Check sheet for the modelled part. Datum: model origin and axes. Units: mm. Face numbers are marked on the shaded views. A direction names the side the tool comes from. Give positions to 0.01 mm unless a question says otherwise; leave off trailing zeros. Order: outer loops, then holes, each group sorted by start corner. A loop starts at its lowest first (then second) coordinate and runs counter-clockwise, first axis right, second up.
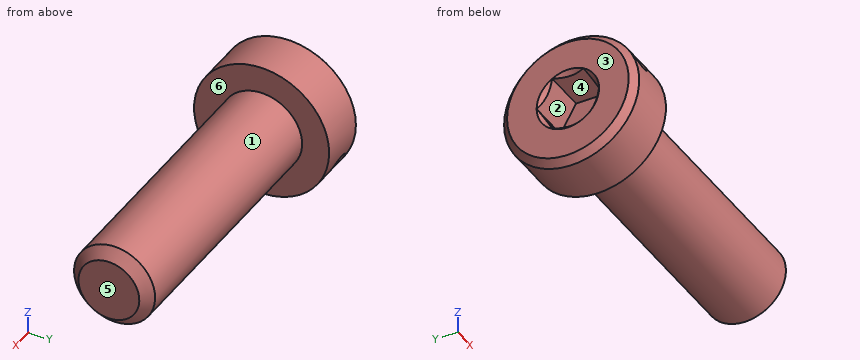
from build123d import *

# Parameters (mm, degrees)
SKETCH2_R               = 3
BOSS_EXTRUDE1_DEPTH     = 20
CHAMFER1_SIZE           = 0.75
CUT_EXTRUDE1_DEPTH      = 3.12
CUT_EXTRUDE3_DEPTH      = 17.652942925
CUT_EXTRUDE3_DEPTH_BACK = 17.652942925
SKETCH9_R               = 0.79375


with BuildPart() as part:
    # Sketch2 → Boss-Extrude1 (new body)
    with BuildSketch(Plane(origin=(10, 0, 0), x_dir=(0, 0, -1), z_dir=(1, 0, 0))):
        Circle(SKETCH2_R)
    extrude(amount=-BOSS_EXTRUDE1_DEPTH)

    # Chamfer1
    chamfer1_edges = [part.edges().sort_by_distance(p)[0] for p in [
        (10, 0, 3),
    ]]
    chamfer(chamfer1_edges, length=CHAMFER1_SIZE)

    # Sketch6 → Revolve1 (revolve)
    with BuildSketch(Plane.XY):
        Polygon((-13.5, 5), (-14, 4.5), (-14, 0), (-10, 0), (-10, 5), align=None)
    revolve(axis=Axis((-10, 0, 0), (-1, 0, 0)))

    # Sketch4 → Cut-Extrude1 (cut)
    with BuildSketch(Plane(origin=(-14, 0, 0), x_dir=(0, 0, -1), z_dir=(1, 0, 0))):
        Polygon((0, 2.309401077), (-2, 1.154700538), (-2, -1.154700538), (0, -2.309401077), (2, -1.154700538), (2, 1.154700538), align=None)
    extrude(amount=CUT_EXTRUDE1_DEPTH, mode=Mode.SUBTRACT)

    # Cut-Extrude2 cone 1 section (through the dimple's axis) → Cut-Extrude2 (revolve, cut)
    with BuildSketch(Plane(origin=(-14, 0, 0), x_dir=(0, 0, 1), z_dir=(0, 1, 0))):
        Polygon((0, 0), (2.309401077, 0), (0, 2.309401077), align=None)
    revolve(axis=Axis((-14, 0, 0), (1, 0, 0)), mode=Mode.SUBTRACT)

    # Sketch9 → Cut-Extrude3 (cut, two sides: drawn at the far end of the back side and taken through both)
    with BuildSketch(Plane(origin=(0, -1.732050808, 1), x_dir=(1, 0, 0), z_dir=(0, 0.8660254037844387, -0.49999999999999983)).offset(-CUT_EXTRUDE3_DEPTH_BACK)):
        with Locations(Location((-12.285299496, 0, 0), (0, 0, 270))):
            Circle(SKETCH9_R)
    extrude(amount=CUT_EXTRUDE3_DEPTH + CUT_EXTRUDE3_DEPTH_BACK, mode=Mode.SUBTRACT)


solid = part.part
1) Depth check by flat-ended pin: pin 1 Ø1.2 at (y, z) = (-1, 0.5) entering from -X; pin 2 Ø2 at (x, y) = (5, -2.5) entering from -Z; pin 3 Ø2 at (x, z) = (-4.5, 3) entering from +Y. Enter the tip coordinate at first touch or a pass-through.
Recorded:
pin 1: stops at x = -10.88
pin 2: stops at z = -2.6
pin 3: stops at y = 2.24
2) Section check B-B, the plane x = -5.75. Record the cut outline in (y, z).
Recorded:
outline: circle Ø6 at (0, 0)
3) Section check A-A, the plane y = 0. Record the cut outline in (x, z).
Recorded:
outline: (-14, -4.5) - (-13.5, -5) - (-10, -5) - (-10, -3) - (9.25, -3) - (10, -2.25) - (10, 2.25) - (9.25, 3) - (-10, 3) - (-10, 5) - (-13.5, 5) - (-14, 4.5) - (-14, 2.31) - (-13.69, 2) - (-10.88, 2) - (-10.88, -2) - (-13.69, -2) - (-14, -2.31) - close
4) Set-up check for the marked faces 5 and 6: record each of +Z, -Z, +X, -X, +Y, -Y from which the full face is reachable in a straight line by a thin tool's end or side.
Recorded:
face 5: +Z, -Z, +X, +Y, -Y
face 6: +X
5) Material ranges on L1, parallel to X at y = 1.75, z = 0.5; L2, parallel to Z at x = -11, y = 2.25; L3, parallel to X at y = -3.5, z = 2.25, recorded low to high.
Recorded:
L1: x = -10.88 to 10
L2: z = -4.47 to -0.1, 0.1 to 4.47
L3: x = -14 to -13.05, -11.52 to -10
6) Draft check along Z on the marked faces 1, 2, 3 and 4. Enter one of: +Z half, -Z half, draft (parallel to the pull), parting line (faces both ways), or undercut.
Recorded:
face 1: parting line
face 2: undercut
face 3: draft
face 4: undercut
